Autodesk Inventor part; units mm, degrees
ref_plane "YZ Plane" through (0, 0, 0) normal (1, 0, 0) x (0, 1, 0)
ref_plane "XZ Plane" through (0, 0, 0) normal (0, 1, 0) x (-1, 0, 0)
ref_plane "XY Plane" through (0, 0, 0) normal (0, 0, 1) x (1, 0, 0)
sketch "Szkic1" plane through (0, 0, 0) normal (0, 1, 0) x (-1, 0, 0)
  circle A0 centre (0, 0) radius 4
  dimension "d0" = 8
extrude "Wyciągnięcie proste1" add sketch "Szkic1" along normal mid plane 35
sketch "Szkic2" plane through (0, 17.5, 0) normal (0, 1, 0) x (1, 0, 0)
  circle A0 centre (0, 0) radius 2.6
  dimension "d3" = 5.2
extrude "Wyciągnięcie proste2" cut sketch "Szkic2" against normal blind 25
thread "Gwint1"
sketch "Szkic3" plane through (0, -17.5, 0) normal (0, -1, 0) x (1, 0, 0)
  line L0 (3.4641, 6) -> (6.9282, 0)
  line L1 (6.9282, 0) -> (3.4641, -6)
  line L2 (3.4641, -6) -> (-3.4641, -6)
  line L3 (-3.4641, -6) -> (-6.9282, 0)
  line L4 (-6.9282, 0) -> (-3.4641, 6)
  line L5 (-3.4641, 6) -> (3.4641, 6)
  point P0 (0, 0)
  point P1 (0, 0)
  dimension "d8" = 6
  dimension "d10" = 6
extrude "Wyciągnięcie proste3" add sketch "Szkic3" along normal blind 5
fillet "Zaokrąglenie1" radius 2 1 edges at (4, -17.5, 0)
properties part number "zamkniecie_sworzenia_2"
Could you check a few things on this model? Use its own coordinates, in mm. A direction names the side the tool comes from. Round coordinates to 2 decimals unless told otherwise and drop trailing zeros. Order: outer loops, then holes, each group sorted by start corner. A loop starts at its lowest first (then second) coordinate and runs counter-clockwise, first axis right, second up. Notation, with made-up numbers: M 39,50 L 72,50 A21 cw 72,60 Z; hole C -3,11 d3. An arc over 180 degrees is marked long. One line per item, written item: value.
(1) If we mould it in two halves opening along X, with no side actions, what happens to faces 3 (the flat face through (-3, 17.5, 0)), 4 (the cylindrical face through (-0.338, 5.175, -2.578)), 5 (the flat face through (5.172, -19.965, 3.042))? For each: released by +X, released by -X, zero draft, split by the parting line, or undercut.
Ans:
face 3: zero draft
face 4: undercut
face 5: released by +X
(2) Imagine slicing it at B-B (y = 5). Write out the boundary of the cut face in (x, z).
Ans:
outline: C 0,0 d8; hole C 0,0 d5.2
(3) I'm going to push flat-ended pins straight in: P1, Ø2, axis at y = 3.5, z = 3.5, coming from the -X side; P2, Ø8, axis at x = 4.5, y = 1.5, coming from the -Z side; P3, Ø3, axis at x = 0, z = 0, coming from the +Y side. Where does each tip first touch, or does it pass through?
Ans:
P1: stops at x = -3.12
P2: stops at z = -3.97
P3: stops at y = -7.5
(4) I need wall thicknesses on line 1 along Z through (x, y) = (0, 8); line 2 along Y through (x, z) = (-1.25, 0.75); line 3 along Y through (x, z) = (4.75, 3.5). Which ranges of each line are inside material? Lowest first, please. Write a range as from..to.
Ans:
line 1: z = -4..-2.6, 2.6..4
line 2: y = -22.5..-7.5
line 3: y = -22.5..-17.5
(5) Which directions (+Z, -Z, +X, -X, +Y, -Y) give clear straight access to the entire face, cutting with the end or side of a thin tool? Please do faces 1 (the flat face through (0, -20, -6)), 2 (the cylindrical face through (0.867, 1.231, -3.905)).
Ans:
face 1: -Z, +X, -X, +Y, -Y
face 2: +Y
